The listing builds one solid part. Answer for the finished solid, in the listing's coordinates (mm). A direction names the side the tool comes from. Give positions to 0.01 mm unless a question says otherwise; leave off trailing zeros. Order: outer loops, then holes, each group sorted by start corner. A loop starts at its lowest first (then second) coordinate and runs counter-clockwise, first axis right, second up. Notation, with made-up numbers: (-12, 9.25) - (30, 9.25) arc R15 cw to (30, 23.25) - close; hole circle Ø11 at (-38, 51). An arc over 180 degrees is marked (long way). Use CSV: the item, a comma, the result in double quotes.
```python
from build123d import *


with BuildPart() as part:
    # Sketch1 → Revolve1 (revolve)
    with BuildSketch(Plane.XY, mode=Mode.PRIVATE) as revolve1_sk:
        Polygon((0, 0), (8, 0), (8, 3.7), (6, 3.7), (6, 9.3), (8, 9.3), (8, 12.3), (4.5, 12.3), (4.5, 14.5), (8, 14.5), (8, 16.1), (4.5, 16.1), (4.5, 18.3), (12.5, 18.3), (12.5, 19.5), (4.5, 19.5), (4.5, 21.7), (12.5, 21.7), (12.5, 22.9), (4.5, 22.9), (4.5, 25.1), (12.5, 25.1), (12.5, 26.3), (4.5, 26.3), (4.5, 28.5), (12.5, 28.5), (12.5, 29.7), (6.5, 29.7), (6.5, 31.9), (12.5, 31.9), (12.5, 33.1), (7.5, 33.1), (7.5, 35.3), (12.5, 35.3), (12.5, 36.5), (7.5, 36.5), (7.5, 38.7), (12.5, 38.7), (12.5, 39.9), (7.5, 39.9), (7.5, 42.1), (12.5, 42.1), (12.5, 43.3), (7.5, 43.3), (7.5, 45.5), (12.5, 45.5), (12.5, 46.7), (7.5, 46.7), (7.5, 48.9), (12.5, 48.9), (12.5, 50.1), (9.200701829, 50.1), (0, 50.1), align=None)
    revolve(revolve1_sk.sketch.rotate(Axis((0, 50.1, 0), (0, -1, 0)), 90), axis=Axis((0, 50.1, 0), (0, -1, 0)))

    # Sketch2 → Cut-Revolve2 (revolve, cut)
    with BuildSketch(Plane.XY, mode=Mode.PRIVATE) as cut_revolve2_sk:
        Polygon((3.2, 0), (3.2, 10), (1.872094381, 12.3), (1.872094381, 18.3), (1, 19.5), (1, 32.1), (1.9, 32.1), (3, 32.735085296), (3, 50.1), (0, 50.1), (0, 0), align=None)
    revolve(cut_revolve2_sk.sketch.rotate(Axis((0, 50.1, 0), (0, -1, 0)), 90), axis=Axis((0, 50.1, 0), (0, -1, 0)), mode=Mode.SUBTRACT)


solid = part.part
```
Item 1: The mould has two halves that part along X. Classify faces 5 (the face through (1, 26, 0)), 6 (the face through (3.4, 14.5, -3.4)), 7 (the face through (7.81, 1.88, -1.73)): +X half, -X half, draft (parallel to the pull), parting line (faces both ways), or undercut.
Taken from the geometry:
face 5,"undercut"
face 6,"draft"
face 7,"parting line"
Item 2: Which of the six approach directions +Z, -Z, +X, -X, +Y, -Y give full straight-line access (tool end or side, diameter ignored) to faces 1 (the face through (8, 43.3, 0)), 2 (the face through (-3.755, 42.708, 11.923)), 3 (the face through (1, 32.1, -1)), 4 (the face through (7.81, 10.82, -1.73))?
Taken from the geometry:
face 1,"none"
face 2,"+Y, -Y"
face 3,"+Y"
face 4,"-Y"
Item 3: Each of these flat-tipped pins is pushed along its axis until it touches: pin 1 (4 mm diameter, centred on x = -0.5, z = -0.5, fed in from +Y); pin 2 (6 mm diameter, centred on y = 37.5, z = 7, fed in from +X); pin 3 (6 mm diameter, centred on y = 24.5, z = 7, fed in from -X); pin 4 (1 mm diameter, centred on y = 7.5, z = 8.5, fed in from +X). Where does it stop, or does it pass through?
Taken from the geometry:
pin 1,"y = 32.57"
pin 2,"x = 11.78"
pin 3,"x = -11.82"
pin 4,"through"
Item 4: The part is cut by section B-B (z = 10.5). Count the separate pieces of the cut face and the enclosed holes in it, and give its area (3 significant figures).
Taken from the geometry:
separate pieces,"10"
enclosed holes,"0"
area,"163 mm^2"
Item 5: The part is cut by section A-A (y = 4.5). Give the vertices of the cut face in (x, z), and give its area (3 significant figures).
Taken from the geometry:
outline,"circle Ø12 at (0, 0); hole circle Ø6.4 at (0, 0)"
area,"80.9 mm^2"
Item 6: Find the intervals of material crossed by line 1 along Y through (x, z) = (-2.5, 4.5); line 2 along X through (y, z) = (3.5, 0); line 3 along X through (y, z) = (6.25, 0), in increasing order.
Taken from the geometry:
line 1,"0 to 12.3, 14.5 to 16.1, 18.3 to 19.5, 21.7 to 22.9, 25.1 to 26.3, 28.5 to 50.1"
line 2,"-8 to -3.2, 3.2 to 8"
line 3,"-6 to -3.2, 3.2 to 6"
Item 7: The part is cut by section D-D (y = 20). Give the vertices of the cut face in (x, z).
Taken from the geometry:
outline,"circle Ø9 at (0, 0); hole circle Ø2 at (0, 0)"
